Autodesk Inventor part; units mm, degrees
ref_plane "Work Plane7" through (0, -46.2947, -99.445) normal (0, -0.9997, 0.0235) x (0, -0.0235, -0.9997)
ref_plane "Work Plane8" through (0, 70.92, -98.723) normal (0, -0.9994, -0.036) x (0, 0.036, -0.9994)
ref_plane "Work Plane9" through (-30, 0, 0) normal (1, 0, 0) x (0, 1, 0)
sketch "Sketch20" plane through (0, 0, 0) normal (1, 0, 0) x (0, 1, 0)
  line L0 (-87.4, 0) -> (69.4, 0)
  line L1 (0, -124.4) -> (0, 74.4) construction
  circle A0 centre (0, 0) radius 40
  circle A1 centre (0, 0) radius 46
  line L2 (35, -29.8496) -> (35, -66)
  line L3 (-35, -66) -> (-35, -29.8496)
  line L4 (47, -66) -> (-65, -66)
  line L5 (47, -66) -> (47, -96)
  line L6 (47, -96) -> (-65, -96)
  line L7 (-65, -96) -> (-65, -66)
  point P0 (0, -66)
  dimension "d254" = 92
  dimension "d255" = 80
  dimension "d256" = 70
  dimension "d261" = 90
  dimension "d262" = 30
  dimension "d263" = 47
  dimension "d264" = 65
  dimension "d265" = 96
  dimension "d268" = 30
  dimension "d269" = 12
  dimension "d273" = 36.1504
extrude "Extrusion18" add sketch "Sketch20" along normal mid plane 60 contours L2 L4 L3 A1 | L4 L5 L6 L7
sketch "Sketch21" plane through (-30, 47, -66) normal (0, 1, 0) x (1, 0, 0)
  line L0 (0, 0) -> (60, 0)
  line L1 (60, 30) -> (60, 0)
  line L2 (0, 30) -> (60, 30)
  line L3 (0, 0) -> (0, 30)
  line L4 (60, 30) -> (60, 0)
  line L5 (0, 0) -> (0, 30)
  arc A0 (60, 1029.0992) -> (0, 1029.0992) centre (30, 530) ccw
  line L6 (0, 30) -> (60, 30)
  point P0 (30, 30)
  point P1 (60, 29.0992)
  point P2 (0, 29.0992)
  dimension "d270" = 500
sketch3d "3D Sketch1"
properties part number "shank_2"
Source: CAD feature listing. Evaluate the final solid. Frame: model axes, mm. A direction names the side the tool comes from. Round coordinates to 2 decimals unless told otherwise and drop trailing zeros. Write each loop counter-clockwise with the first axis right and the second up, starting at its lowest first coordinate (ties: lowest second). Pieces come first, ordered by that corner, then holes. Notation, with made-up numbers: M 17,46.25 L 39,46.25 A27 cw 39,64.25 Z; hole C 29,87 d7. An arc over 180 degrees is marked long. Use CSV: the item, a comma, the result in double quotes. Start each with the question number.
Q1. Cut plane A-A on x = 13. Output: boundary loops of the cut face in (y, z).
Q2. First-contact query: P1, Ø15, axis at x = 0.5, y = -47.5, coming from the +Z side; P2, Ø4, axis at x = -5.5, z = -51.5, coming from the -Y side; P3, Ø11, axis at x = 4.5, z = -44.5, coming from the +Y side. Flat tips, straight axial feed; report the tip coordinate or a pass-through.
Q3. Access query for faces 1 (the face through (0, -8, -96)), 2 (the face through (0, -50, -66)), 3 (the face through (0, 35, -48)). Directions: +Z, -Z, +X, -X, +Y, -Y. A direction counts if a zero-diameter tool reaches every point of the face in a straight line with its end or side. Return the directions, or none.
Q4. Line query: line 1 (Y direction, x = 11, z = -35); line 2 (Z direction, x = -4, y = 36); line 3 (Y direction, x = -18, z = -37). Output: solid intervals per line, ascending. Write a range as from..to.
Q5. Cut plane B-B on z = -40. Output: boundary loops of the cut face in (x, y), plus the area to 3 significant figures.
Q6. Cut plane D-D on y = 10. Output: boundary loops of the cut face in (x, z), plus the area to 3 significant figures.
Q7. Cut plane C-C on z = -53. Output: boundary loops of the cut face in (x, y).
Results found:
1,outline,"M -65,-96 L 47,-96 L 47,-66 L 35,-66 L 35,-29.85 A46 cw -35,-29.85 L -35,-66 L -65,-66 Z"
2,P1,"z = -66"
2,P2,"y = -35"
2,P3,"y = 35"
3,face 1,"-Z, +X, -X, +Y, -Y"
3,face 2,"+Z, +X, -X, -Y"
3,face 3,"+Z, +X, -X, +Y"
4,line 1,"-35..-29.85, 29.85..35"
4,line 2,"-96..-66"
4,line 3,"-35..-27.33, 27.33..35"
5,outline,"M -30,-35 L 30,-35 L 30,-22.72 L -30,-22.72 Z; M -30,22.72 L 30,22.72 L 30,35 L -30,35 Z"
5,area,"1,470 mm^2"
6,outline,"M -30,-96 L 30,-96 L 30,-44.9 L -30,-44.9 Z"
6,area,"3,070 mm^2"
7,outline,"M -30,-35 L 30,-35 L 30,35 L -30,35 Z"
